Design review of the part built by this model. Coordinates are the model's own, in mm. A direction names the side the tool comes from. Coordinates: 2 decimals unless noted, no trailing zeros. Loops run counter-clockwise (first coordinate to the right, second up) from the corner with the lowest first, then second, coordinate; pieces in that order, holes last.
from build123d import *

# Parameters (mm, degrees)
F0_W            = 240
F0_H            = 50
F1_DEPTH        = 63.5
F3_DEPTH        = 63.501
F4_R            = 22.5
F5_DEPTH        = 5
F6_R            = 22.5
F7_DEPTH        = 5
F8_W            = 33.4643870592
F8_H            = 0.5
F8_W_2          = 31.9364720583
F9_DEPTH        = 63.501
F11_D           = 8.8
F11_DEPTH       = 35
F11_CBORE_D     = 10
F11_CBORE_DEPTH = 25
F11_TIP         = 2.6437867237
F12_W           = 154
F12_H           = 30
F13_DEPTH       = 132
F15_DEPTH       = 63.501
F16_W           = 1
F16_H           = 104.974
F17_DEPTH       = 46.751
F18_W           = 40
F18_H           = 35
F19_DEPTH       = 46.751
F21_D           = 8.8
F21_DEPTH       = 93
F21_TIP         = 2.6437867237


with BuildPart() as f1:
    # F0 (on Front) → F1 (new body)
    with BuildSketch(Plane.XZ):
        with Locations((120, 25)):
            Rectangle(F0_W, F0_H)
    extrude(amount=F1_DEPTH)

    # F2 (on face) → F3 (cut, through all)
    with BuildSketch(Plane.XZ.offset(63.5)):
        with BuildLine():
            Line((22.5, 25), (40, 25))
            Line((40, 25), (57.5, 25))
            ThreePointArc((57.5, 25), (40, 42.5), (22.5, 25))
        make_face()
        with BuildLine():
            Line((57.5, 25), (40, 25))
            Line((40, 25), (22.5, 25))
            ThreePointArc((22.5, 25), (40, 7.5), (57.5, 25))
        make_face()
        with BuildLine():
            ThreePointArc((217.5, 25), (200, 42.5), (182.5, 25))
            Line((182.5, 25), (200, 25))
            Line((200, 25), (217.5, 25))
        make_face()
        with BuildLine():
            Line((200, 25), (182.5, 25))
            ThreePointArc((182.5, 25), (200, 7.5), (217.5, 25))
            Line((217.5, 25), (200, 25))
        make_face()
        with BuildLine():
            ThreePointArc((120, 40), (109.3933982822, 35.6066017178), (105, 25))
            Line((105, 25), (120, 25))
            Line((120, 25), (120, 40))
        make_face()
        with BuildLine():
            Line((120, 25), (105, 25))
            ThreePointArc((105, 25), (109.3933982822, 14.3933982822), (120, 10))
            Line((120, 10), (120, 25))
        make_face()
        with BuildLine():
            Line((120, 40), (120, 25))
            Line((120, 25), (135, 25))
            ThreePointArc((135, 25), (130.6066017178, 35.6066017178), (120, 40))
        make_face()
        with BuildLine():
            Line((135, 25), (120, 25))
            Line((120, 25), (120, 10))
            ThreePointArc((120, 10), (130.6066017178, 14.3933982822), (135, 25))
        make_face()
    extrude(amount=-F3_DEPTH, mode=Mode.SUBTRACT)

    # F4 (on face) → F5 (cut)
    with BuildSketch(Plane.XZ.offset(63.5)):
        with Locations((120, 25)):
            Circle(F4_R)
    extrude(amount=-F5_DEPTH, mode=Mode.SUBTRACT)

    # F6 (on face) → F7 (cut)
    with BuildSketch(Plane(origin=(0, 0, 0), x_dir=(-1, 0, 0), z_dir=(0, 1, 0))):
        with Locations((-120, 25)):
            Circle(F6_R)
    extrude(amount=-F7_DEPTH, mode=Mode.SUBTRACT)

    # F8 (on face) → F9 (cut, through all)
    with BuildSketch(Plane.XZ.offset(63.5)):
        with Locations((16.7321935296, 25.25)):
            Rectangle(F8_W, F8_H)
        with Locations((16.7321935296, 24.75)):
            Rectangle(F8_W, F8_H)
        with Locations((224.0317639709, 24.75)):
            Rectangle(F8_W_2, F8_H)
        with Locations((224.0317639709, 25.25)):
            Rectangle(F8_W_2, F8_H)
    extrude(amount=-F9_DEPTH, mode=Mode.SUBTRACT)

    # F11
    with Locations(Plane.XY.offset(50)):
        with Locations((11, -20), (11, -43.5), (229, -20), (229, -43.5)):
            CounterBoreHole(F11_D / 2, F11_CBORE_D / 2, F11_CBORE_DEPTH, depth=F11_DEPTH)
            with Locations((0, 0, -(F11_DEPTH + F11_TIP / 2))):  # 118° drill point
                Cone(0, F11_D / 2, F11_TIP, mode=Mode.SUBTRACT)

    # F12 (on face) → F13 (join)
    with BuildSketch(Plane.XY.offset(50)):
        with Locations((120, -31.75)):
            Rectangle(F12_W, F12_H)
    extrude(amount=F13_DEPTH)

    # F14 (on face) → F15 (cut, through all)
    with BuildSketch(Plane.XZ.offset(63.5)):
        with BuildLine():
            ThreePointArc((120, 68), (141.9203102168, 77.0796897832), (151, 99))
            ThreePointArc((151, 99), (98.0796897832, 120.9203102168), (120, 68))
        make_face()
        with BuildLine():
            ThreePointArc((151, 99), (98.0796897832, 120.9203102168), (120, 68))
            ThreePointArc((120, 68), (141.9203102168, 77.0796897832), (151, 99))
        make_face()
    extrude(amount=-F15_DEPTH, mode=Mode.SUBTRACT)

    # F16 (on face) → F17 (cut, through all)
    with BuildSketch(Plane.XZ.offset(46.75)):
        with Locations((119.5, 151.487)):
            Rectangle(F16_W, F16_H)
        with Locations((120.5, 151.487)):
            Rectangle(F16_W, F16_H)
    extrude(amount=-F17_DEPTH, mode=Mode.SUBTRACT)

    # F18 (on face) → F19 (cut, through all)
    with BuildSketch(Plane.XZ.offset(46.75)):
        with Locations((63, 164.5)):
            Rectangle(F18_W, F18_H)
        with Locations((177, 164.5)):
            Rectangle(F18_W, F18_H)
    extrude(amount=-F19_DEPTH, mode=Mode.SUBTRACT)

    # F21
    with Locations(Plane(origin=(83, 0, 0), x_dir=(0, -1, 0), z_dir=(-1, 0, 0))):
        with Locations((31.75, 160.9999984503)):
            Hole(F21_D / 2, depth=F21_DEPTH)
            with Locations((0, 0, -(F21_DEPTH + F21_TIP / 2))):  # 118° drill point
                Cone(0, F21_D / 2, F21_TIP, mode=Mode.SUBTRACT)


solid = f1.part
Q1. Take a section at A-A, the plane x = 200. Write out the cut boundary in (y, z).
Q2. Take a section at B-B, the plane z = 150.5. Write out the cut boundary in (x, y).
Q3. Machinability: for faces 1 (the flat face through (11, -32, 25.5)), 2 (the cylindrical face through (102.145, -61.035, 11.309)), 3 (the flat face through (136, -16.75, 130)), 4 (the flat face through (105, -5, 20)), 5 (the cylindrical face through (233.77, -42, 37.92)), which of the approach directions +Z, -Z, +X, -X, +Y, -Y give a long, thin tool a straight path to every point of the face, cutting with its end or side? Answer none if there is none.
Q4. Take a section at D-D, the plane y = -31.75. Give the number of separate pieces and of enclosed holes in the cut face, then the cut area to 3 significant figures.
Q5. The part is to be moulded in two halves that separate along X. For faces 6 (the flat face through (0, -31, 38)), 7 (the cylindrical face through (233.77, -18.5, 37.92)), 8 (the cylindrical face through (137.855, -2.465, 11.309)), 9 (the flat face through (136, -46.75, 130)), say which applies: pulls with the +X half, pulls with the -X half, needs draft (parallel to the pull), parting line crosses it, or undercut.
Q6. Clearance check with flat-ended pins moving along their axes: pin 1 Ø3 at (y, z) = (-41.5, 144.5) entering from +X; pin 2 Ø15 at (y, z) = (-36.5, 157) entering from -X; pin 3 Ø8 at (x, y) = (229, -20) entering from +Z. State where each tip first meets the part, or that it passes through.
Q7. Take a section at C-C, the plane z = 30.5. Write out the cut boundary in (x, y).
Q8. For line 1 (Y direction, x = 229, z = 22); line 2 (Y direction, x = 229, z = 33.25); line 3 (X direction, y = -53.5, z = 21.5), list the stretches that pass through material, from the lowest coordinate up.
Entries:
1. outline: (-63.5, 0) - (0, 0) - (0, 7.5) - (-63.5, 7.5) - close; (-63.5, 42.5) - (0, 42.5) - (0, 50) - (-63.5, 50) - close
2. outline: (83, -46.75) - (119, -46.75) - (119, -16.75) - (83, -16.75) - close; (121, -46.75) - (157, -46.75) - (157, -16.75) - (121, -16.75) - close
3. face 1: -X, +Y, -Y
3. face 2: -Y
3. face 3: +Z, +X, -X, +Y
3. face 4: +Y
3. face 5: +Z
4. separate pieces: 3
4. enclosed holes: 1
4. area: 23,100 mm2
5. face 6: pulls with the -X half
5. face 7: undercut
5. face 8: undercut
5. face 9: needs draft
6. pin 1: stops at x = 197
6. pin 2: stops at x = 83
6. pin 3: stops at z = 14.76
7. outline: (0, -63.5) - (23.39, -63.5) - (23.39, 0) - (0, 0) - close; (56.61, -63.5) - (98.18, -63.5) - (98.18, -58.5) - (106.04, -58.5) - (106.04, -5) - (98.18, -5) - (98.18, 0) - (56.61, 0) - close; (133.96, -58.5) - (141.82, -58.5) - (141.82, -63.5) - (183.39, -63.5) - (183.39, 0) - (141.82, 0) - (141.82, -5) - (133.96, -5) - close; (216.61, -63.5) - (240, -63.5) - (240, 0) - (216.61, 0) - close; hole circle Ø10 at (11, -43.5); hole circle Ø10 at (11, -20); hole circle Ø10 at (229, -43.5); hole circle Ø10 at (229, -20)
8. line 1: y = -63.5 to -47.9, -39.1 to -24.4, -15.6 to 0
8. line 2: y = -63.5 to -48.5, -38.5 to -25, -15 to 0
8. line 3: x = 0 to 22.85, 57.15 to 105.41, 134.59 to 182.85, 217.15 to 240
